from build123d import *

# Parameters (mm, degrees)
SKETCH1_W                                           = 120
SKETCH1_H                                           = 70
BOSS_EXTRUDE1_DEPTH                                 = 2.5
FILLET1_R                                           = 2
CSK_FOR_M3_COUNTERSUNK_FLAT_HEAD_SCREW1_D           = 3.4
CSK_FOR_M3_COUNTERSUNK_FLAT_HEAD_SCREW1_DEPTH       = 10
CSK_FOR_M3_COUNTERSUNK_FLAT_HEAD_SCREW1_CSINK_D     = 6.3
CSK_FOR_M3_COUNTERSUNK_FLAT_HEAD_SCREW1_CSINK_ANGLE = 90
CSK_FOR_M3_COUNTERSUNK_FLAT_HEAD_SCREW1_TIP         = 1.021463052
FILLET2_R                                           = 0.5


with BuildPart() as part:
    # Sketch1 → Boss-Extrude1 (new body)
    with BuildSketch(Plane.XY):
        Rectangle(SKETCH1_W, SKETCH1_H)
    extrude(amount=BOSS_EXTRUDE1_DEPTH)

    # Fillet1
    fillet1_edges = [part.edges().sort_by_distance(p)[0] for p in [
        (-60, 35, 1.25),
        (60, 35, 1.25),
        (60, -35, 1.25),
        (-60, -35, 1.25),
    ]]
    fillet(fillet1_edges, radius=FILLET1_R)

    # CSK for M3 Countersunk Flat Head Screw1
    with Locations(Plane(origin=(-55.8, 30.8, 2.5), x_dir=(1, 0, 0), z_dir=(0, 0, 1))):
        with Locations((0, 0), (111.6, 0), (111.6, -61.6), (0, -61.6)):
            CounterSinkHole(CSK_FOR_M3_COUNTERSUNK_FLAT_HEAD_SCREW1_D / 2, CSK_FOR_M3_COUNTERSUNK_FLAT_HEAD_SCREW1_CSINK_D / 2, depth=CSK_FOR_M3_COUNTERSUNK_FLAT_HEAD_SCREW1_DEPTH, counter_sink_angle=CSK_FOR_M3_COUNTERSUNK_FLAT_HEAD_SCREW1_CSINK_ANGLE)
            with Locations((0, 0, -(CSK_FOR_M3_COUNTERSUNK_FLAT_HEAD_SCREW1_DEPTH + CSK_FOR_M3_COUNTERSUNK_FLAT_HEAD_SCREW1_TIP / 2))):  # 118° drill point
                Cone(0, CSK_FOR_M3_COUNTERSUNK_FLAT_HEAD_SCREW1_D / 2, CSK_FOR_M3_COUNTERSUNK_FLAT_HEAD_SCREW1_TIP, mode=Mode.SUBTRACT)

    # Fillet2
    fillet2_edges = [part.edges().sort_by_distance(p)[0] for p in [
        (60, 0, 2.5),
        (0, -35, 2.5),
        (-60, 0, 2.5),
        (0, 35, 2.5),
        (59.414213562, 34.414213562, 2.5),
        (-59.414213562, 34.414213562, 2.5),
        (-59.414213562, -34.414213562, 2.5),
        (59.414213562, -34.414213562, 2.5),
    ]]
    fillet(fillet2_edges, radius=FILLET2_R)


solid = part.part
Build history of the part. All positions in model axes, mm. Round coordinates to 2 decimals unless told otherwise and drop trailing zeros. Loops run counter-clockwise (first coordinate to the right, second up) from the corner with the lowest first, then second, coordinate; pieces in that order, holes last. Notation, with made-up numbers: (-40, 71) -> (-22, 71) arc R21 ccw to (-22, 103) -> close; hole circle Ø3 at (17.5, 88.5). An arc over 180 degrees is marked (long way). One line per item, written item: value. Start each with the question number.
Q1. Probe line 1 along X through (y, z) = (30.8, 0.65); line 2 along Y through (x, z) = (-55.8, 0.2); line 3 along X through (y, z) = (-29.5, 1.65). List the from-to ranges inside material, lowest first.
Q2. Cut at B-B on y = -30.8. List the corners of the cut face in (x, z).
Q3. Cut at A-A on x = -55.8. List the corners of the cut face in (y, z).
Q4. Drop flat-ended pins along their axis: pin 1 Ø1.5 at (x, y) = (37.5, 24.5) entering from -Z; pin 2 Ø4 at (x, y) = (55.8, -30.8) entering from +Z. Give the stop position or say it passes through.
Q5. Two-plate mould, pull along Y, no slides. Class faces 1 (the face through (57.05, 31.95, 0.52)), 2 (the face through (-1, 0, 2.5)): released by +Y, released by -Y, zero draft, split by the parting line, or undercut.
Computed:
1. line 1: -60 to -57.5, -54.1 to 54.1, 57.5 to 60
1. line 2: -35 to -32.5, -29.1 to 29.1, 32.5 to 35
1. line 3: -60 to -57.7, -53.9 to 53.9, 57.7 to 60
2. outline: (-60, 0) -> (-57.5, 0) -> (-57.5, 1.05) -> (-58.95, 2.5) -> (-59.5, 2.5) arc R0.5 ccw to (-60, 2) -> close; (-54.1, 0) -> (54.1, 0) -> (54.1, 1.05) -> (52.65, 2.5) -> (-52.65, 2.5) -> (-54.1, 1.05) -> close; (57.5, 0) -> (60, 0) -> (60, 2) arc R0.5 ccw to (59.5, 2.5) -> (58.95, 2.5) -> (57.5, 1.05) -> close
3. outline: (-35, 0) -> (-32.5, 0) -> (-32.5, 1.05) -> (-33.95, 2.5) -> (-34.5, 2.5) arc R0.5 ccw to (-35, 2) -> close; (-29.1, 0) -> (29.1, 0) -> (29.1, 1.05) -> (27.65, 2.5) -> (-27.65, 2.5) -> (-29.1, 1.05) -> close; (32.5, 0) -> (35, 0) -> (35, 2) arc R0.5 ccw to (34.5, 2.5) -> (33.95, 2.5) -> (32.5, 1.05) -> close
4. pin 1: z = 0
4. pin 2: z = 1.35
5. face 1: undercut
5. face 2: zero draft
